```python
from build123d import *

# Parameters (mm, degrees)
F1_DEPTH = 2
F2_DEPTH = 15
F3_DEPTH = 6
F4_DEPTH = 23.4


with BuildPart() as f1:
    # F0 (on Top) → F1 (new body)
    with BuildSketch(Plane.XY):
        with BuildLine():
            ThreePointArc((-15.1641591538, -3.2090928871), (-15.5, 0), (-15.1641591538, 3.2090928871))
            Line((-15.1641591538, 3.2090928871), (-18.2195423335, 3.2090928871))
            ThreePointArc((-18.2195423335, 3.2090928871), (-18.5, 0), (-18.2195423335, -3.2090928871))
            Line((-18.2195423335, -3.2090928871), (-15.1641591538, -3.2090928871))
        make_face()
        with BuildLine():
            Line((-18.2195423335, 3.2090928871), (-15.1641591538, 3.2090928871))
            ThreePointArc((-15.1641591538, 3.2090928871), (1.6133091948, 15.415811151), (15.5, 0))
            ThreePointArc((15.5, 0), (1.6133091948, -15.415811151), (-15.1641591538, -3.2090928871))
            Line((-15.1641591538, -3.2090928871), (-18.2195423335, -3.2090928871))
            ThreePointArc((-18.2195423335, -3.2090928871), (1.610662415, -18.4297522117), (18.5, 0))
            ThreePointArc((18.5, 0), (1.610662415, 18.4297522117), (-18.2195423335, 3.2090928871))
        make_face()
    extrude(amount=F1_DEPTH)

    # F0 (on Top) → F2 (join)
    with BuildSketch(Plane.XY):
        with BuildLine():
            ThreePointArc((-12.0810480854, -3.2090928871), (-12.5, 0), (-12.0810480854, 3.2090928871))
            Line((-12.0810480854, 3.2090928871), (-15.1641591538, 3.2090928871))
            ThreePointArc((-15.1641591538, 3.2090928871), (-15.5, 0), (-15.1641591538, -3.2090928871))
            Line((-15.1641591538, -3.2090928871), (-12.0810480854, -3.2090928871))
        make_face()
        with BuildLine():
            Line((-15.1641591538, 3.2090928871), (-12.0810480854, 3.2090928871))
            ThreePointArc((-12.0810480854, 3.2090928871), (1.6181623733, 12.3948195039), (12.5, 0))
            ThreePointArc((12.5, 0), (1.6181623733, -12.3948195039), (-12.0810480854, -3.2090928871))
            Line((-12.0810480854, -3.2090928871), (-15.1641591538, -3.2090928871))
            ThreePointArc((-15.1641591538, -3.2090928871), (1.6133091948, -15.415811151), (15.5, 0))
            ThreePointArc((15.5, 0), (1.6133091948, 15.415811151), (-15.1641591538, 3.2090928871))
        make_face()
    extrude(amount=F2_DEPTH)

    # F0 (on Top) → F3 (join)
    with BuildSketch(Plane.XY):
        with BuildLine():
            ThreePointArc((-5.9951416032, -3.2090928871), (-6.8, 0), (-5.9951416032, 3.2090928871))
            Line((-5.9951416032, 3.2090928871), (-12.0810480854, 3.2090928871))
            ThreePointArc((-12.0810480854, 3.2090928871), (-12.5, 0), (-12.0810480854, -3.2090928871))
            Line((-12.0810480854, -3.2090928871), (-5.9951416032, -3.2090928871))
        make_face()
        with BuildLine():
            ThreePointArc((-5.9951416032, 3.2090928871), (1.6542425908, 6.595716902), (6.8, 0))
            ThreePointArc((6.8, 0), (1.6542425908, -6.595716902), (-5.9951416032, -3.2090928871))
            Line((-5.9951416032, -3.2090928871), (-12.0810480854, -3.2090928871))
            ThreePointArc((-12.0810480854, -3.2090928871), (1.6181623733, -12.3948195039), (12.5, 0))
            ThreePointArc((12.5, 0), (1.6181623733, 12.3948195039), (-12.0810480854, 3.2090928871))
            Line((-12.0810480854, 3.2090928871), (-5.9951416032, 3.2090928871))
        make_face()
    extrude(amount=F3_DEPTH)

    # F0 (on Top) → F4 (cut)
    with BuildSketch(Plane.XY):
        with BuildLine():
            ThreePointArc((-18.2195423335, -3.2090928871), (-18.5, 0), (-18.2195423335, 3.2090928871))
            Line((-18.2195423335, 3.2090928871), (-24.5871795341, 3.2090928871))
            Line((-24.5871795341, 3.2090928871), (-24.5871795341, -3.2090928871))
            Line((-24.5871795341, -3.2090928871), (-18.2195423335, -3.2090928871))
        make_face()
        with BuildLine():
            ThreePointArc((-5.9951416032, -3.2090928871), (-6.8, 0), (-5.9951416032, 3.2090928871))
            Line((-5.9951416032, 3.2090928871), (-12.0810480854, 3.2090928871))
            ThreePointArc((-12.0810480854, 3.2090928871), (-12.5, 0), (-12.0810480854, -3.2090928871))
            Line((-12.0810480854, -3.2090928871), (-5.9951416032, -3.2090928871))
        make_face()
        with BuildLine():
            ThreePointArc((-15.1641591538, -3.2090928871), (-15.5, 0), (-15.1641591538, 3.2090928871))
            Line((-15.1641591538, 3.2090928871), (-18.2195423335, 3.2090928871))
            ThreePointArc((-18.2195423335, 3.2090928871), (-18.5, 0), (-18.2195423335, -3.2090928871))
            Line((-18.2195423335, -3.2090928871), (-15.1641591538, -3.2090928871))
        make_face()
        with BuildLine():
            ThreePointArc((-12.0810480854, -3.2090928871), (-12.5, 0), (-12.0810480854, 3.2090928871))
            Line((-12.0810480854, 3.2090928871), (-15.1641591538, 3.2090928871))
            ThreePointArc((-15.1641591538, 3.2090928871), (-15.5, 0), (-15.1641591538, -3.2090928871))
            Line((-15.1641591538, -3.2090928871), (-12.0810480854, -3.2090928871))
        make_face()
    extrude(amount=F4_DEPTH, mode=Mode.SUBTRACT)


solid = f1.part
```
Source: CAD feature listing. Evaluate the final solid. Frame: model axes, mm. A direction names the side the tool comes from. Give positions to 0.01 mm unless a question says otherwise; leave off trailing zeros. Write each loop counter-clockwise with the first axis right and the second up, starting at its lowest first coordinate (ties: lowest second). Pieces come first, ordered by that corner, then holes.
1. Section query A-A (x = 3.5). Return the cut outline in (y, z).
2. Pull-direction query (Y, two-part tool) for faces 1 (the face through (12.3, 9.7, 2)), 2 (the face through (-12, 3.209, 5.7)); classes: +Y half, -Y half, draft (parallel to the pull), parting line (faces both ways), or undercut.
3. Section query D-D (y = 8.5). Return the cut outline in (x, z), then the cut area to 3 significant figures.
4. Material intervals for line 1 along X through (y, z) = (10, 6.5); line 2 along Y through (x, z) = (-14, 12.75); line 3 along Y through (x, z) = (7.5, 6.25), sorted ascending.
5. Section query C-C (y = 4). Return the cut outline in (x, z), then the cut area to 3 significant figures.
6. Access query for faces 3 (the face through (13, 0, 15)), 4 (the face through (-12.2, -3.209, 5.7)), 5 (the face through (5, -5, 6)). Directions: +Z, -Z, +X, -X, +Y, -Y. A direction counts if a zero-diameter tool reaches every point of the face in a straight line with its end or side. Return the directions, or none.
7. First-contact query: pin 1 (2 mm diameter, centred on x = -10, z = 5, fed in from -Y); pin 2 (8 mm diameter, centred on y = -12.5, z = 9, fed in from +X); pin 3 (5 mm diameter, centred on x = 3, z = 10.5, fed in from -Y). Flat tips, straight axial feed; report the tip coordinate or a pass-through.
8. Section query B-B (z = 11.75). Return the cut outline in (x, y).
Output values:
1. outline: (-18.17, 0) - (-5.83, 0) - (-5.83, 6) - (-12, 6) - (-12, 15) - (-15.1, 15) - (-15.1, 2) - (-18.17, 2) - close; (5.83, 0) - (18.17, 0) - (18.17, 2) - (15.1, 2) - (15.1, 15) - (12, 15) - (12, 6) - (5.83, 6) - close
2. face 1: draft
2. face 2: undercut
3. outline: (-16.43, 0) - (16.43, 0) - (16.43, 2) - (12.96, 2) - (12.96, 15) - (9.17, 15) - (9.17, 6) - (-9.17, 6) - (-9.17, 15) - (-12.96, 15) - (-12.96, 2) - (-16.43, 2) - close
3. area: 238 mm2
4. line 1: x = -11.84 to -7.5, 7.5 to 11.84
4. line 2: y = -6.65 to -3.21, 3.21 to 6.65
4. line 3: y = -13.56 to -10, 10 to 13.56
5. outline: (-18.06, 0) - (-5.5, 0) - (-5.5, 6) - (-11.84, 6) - (-11.84, 15) - (-14.97, 15) - (-14.97, 2) - (-18.06, 2) - close; (5.5, 0) - (18.06, 0) - (18.06, 2) - (14.97, 2) - (14.97, 15) - (11.84, 15) - (11.84, 6) - (5.5, 6) - close
5. area: 182 mm2
6. face 3: +Z, +X, -X, +Y, -Y
6. face 4: +Z, -Z, -X
6. face 5: +Z
7. pin 1: stops at y = -12.62
7. pin 2: stops at x = 12.96
7. pin 3: stops at y = -15.49
8. outline: (-15.16, -3.21) arc R15.5 ccw (long way) to (-15.16, 3.21) - (-12.08, 3.21) arc R12.5 cw (long way) to (-12.08, -3.21) - close
